```python
from build123d import *

# Parameters (mm, degrees)
CYLINDER1887_R     = 5
CYLINDER1887_DEPTH = 5
CYLINDER1886_R     = 2.5
CYLINDER1886_DEPTH = 40
CYLINDER1800_R     = 5
CYLINDER1800_DEPTH = 3
CYLINDER1801_R     = 2.5
CYLINDER1801_DEPTH = 20
CYLINDER1798_R     = 1.5
CYLINDER1798_DEPTH = 20
CYLINDER1796_R     = 1.5
CYLINDER1796_DEPTH = 20
CYLINDER1797_R     = 1.5
CYLINDER1797_DEPTH = 20
CYLINDER1799_R     = 1.5
CYLINDER1799_DEPTH = 20
BOX758_W           = 6
BOX758_H           = 6
BOX758_DEPTH       = 2
BOX760_W           = 6
BOX760_H           = 6
BOX760_DEPTH       = 2
BOX759_W           = 6
BOX759_H           = 6
BOX759_DEPTH       = 2
BOX756_W           = 6
BOX756_H           = 6
BOX756_DEPTH       = 2
BOX757_W           = 20
BOX757_H           = 80
BOX757_DEPTH       = 20
BOX761_W           = 38
BOX761_H           = 32
BOX761_DEPTH       = 26
CHAMFER064_SIZE    = 2


with BuildPart() as obj1:
    # Cylinder1887 → Cylinder1887 (new body)
    with BuildSketch(Plane(origin=(-86, 16, 68), x_dir=(0, 0, -1), z_dir=(1, 0, 0))):
        Circle(CYLINDER1887_R)
    extrude(amount=CYLINDER1887_DEPTH)


with BuildPart() as obj2:
    # Cylinder1886 → Cylinder1886 (new body)
    with BuildSketch(Plane(origin=(-90, 16, 68), x_dir=(0, 0, -1), z_dir=(1, 0, 0))):
        Circle(CYLINDER1886_R)
    extrude(amount=CYLINDER1886_DEPTH)


with BuildPart() as obj3:
    # Cylinder1800 → Cylinder1800 (new body)
    with BuildSketch(Plane(origin=(-112, 16, 66), x_dir=(0, 0, -1), z_dir=(1, 0, 0))):
        Circle(CYLINDER1800_R)
    extrude(amount=CYLINDER1800_DEPTH)


with BuildPart() as obj4:
    # Cylinder1801 → Cylinder1801 (new body)
    with BuildSketch(Plane(origin=(-117, 16, 66), x_dir=(0, 0, -1), z_dir=(1, 0, 0))):
        Circle(CYLINDER1801_R)
    extrude(amount=CYLINDER1801_DEPTH)


with BuildPart() as obj5:
    # Cylinder1798 → Cylinder1798 (new body)
    with BuildSketch(Plane(origin=(-83, 25, 54), x_dir=(1, 0, 0), z_dir=(0, 0, 1))):
        Circle(CYLINDER1798_R)
    extrude(amount=CYLINDER1798_DEPTH)


with BuildPart() as obj6:
    # Cylinder1796 → Cylinder1796 (new body)
    with BuildSketch(Plane(origin=(-109, 7, 54), x_dir=(1, 0, 0), z_dir=(0, 0, 1))):
        Circle(CYLINDER1796_R)
    extrude(amount=CYLINDER1796_DEPTH)


with BuildPart() as obj7:
    # Cylinder1797 → Cylinder1797 (new body)
    with BuildSketch(Plane(origin=(-109, 25, 54), x_dir=(1, 0, 0), z_dir=(0, 0, 1))):
        Circle(CYLINDER1797_R)
    extrude(amount=CYLINDER1797_DEPTH)


with BuildPart() as compound920:
    # Cylinder1799 → Cylinder1799 (new body)
    with BuildSketch(Plane(origin=(-83, 7, 54), x_dir=(1, 0, 0), z_dir=(0, 0, 1))):
        Circle(CYLINDER1799_R)
    extrude(amount=CYLINDER1799_DEPTH)

    # Compound920: union obj5, obj6, obj7
    add(obj5.part)
    add(obj6.part)
    add(obj7.part)


with BuildPart() as krychle758:
    # Box758 → Box758 (new body)
    with BuildSketch(Plane(origin=(-112, 22, 60), x_dir=(1, 0, 0), z_dir=(0, 0, 1))):
        with Locations((3, 3)):
            Rectangle(BOX758_W, BOX758_H)
    extrude(amount=BOX758_DEPTH)


with BuildPart() as krychle760:
    # Box760 → Box760 (new body)
    with BuildSketch(Plane(origin=(-86, 4, 60), x_dir=(1, 0, 0), z_dir=(0, 0, 1))):
        with Locations((3, 3)):
            Rectangle(BOX760_W, BOX760_H)
    extrude(amount=BOX760_DEPTH)


with BuildPart() as krychle759:
    # Box759 → Box759 (new body)
    with BuildSketch(Plane(origin=(-86, 22, 60), x_dir=(1, 0, 0), z_dir=(0, 0, 1))):
        with Locations((3, 3)):
            Rectangle(BOX759_W, BOX759_H)
    extrude(amount=BOX759_DEPTH)


with BuildPart() as compound918:
    # Box756 → Box756 (new body)
    with BuildSketch(Plane(origin=(-112, 4, 60), x_dir=(1, 0, 0), z_dir=(0, 0, 1))):
        with Locations((3, 3)):
            Rectangle(BOX756_W, BOX756_H)
    extrude(amount=BOX756_DEPTH)

    # Compound918: union Krychle758, Krychle760, Krychle759
    add(krychle758.part)
    add(krychle760.part)
    add(krychle759.part)


with BuildPart() as krychle757:
    # Box757 → Box757 (new body)
    with BuildSketch(Plane(origin=(-106, 4, 56), x_dir=(1, 0, 0), z_dir=(0, 0, 1))):
        with Locations((10, 40)):
            Rectangle(BOX757_W, BOX757_H)
    extrude(amount=BOX757_DEPTH)


with BuildPart() as cut620:
    # Box761 → Box761 (new body)
    with BuildSketch(Plane(origin=(-112, 0, 56), x_dir=(1, 0, 0), z_dir=(0, 0, 1))):
        with Locations((19, 16)):
            Rectangle(BOX761_W, BOX761_H)
    extrude(amount=BOX761_DEPTH)

    # Cut567: cut Krychle757
    add(krychle757.part, mode=Mode.SUBTRACT)

    # Cut569: cut Compound918
    add(compound918.part, mode=Mode.SUBTRACT)

    # Cut563: cut Compound920
    add(compound920.part, mode=Mode.SUBTRACT)

    # Cut564: cut obj4
    add(obj4.part, mode=Mode.SUBTRACT)

    # Cut560: cut obj3
    add(obj3.part, mode=Mode.SUBTRACT)

    # Chamfer064
    chamfer064_edges = [cut620.edges().sort_by_distance(p)[0] for p in [
        (-112, 32, 69),
    ]]
    chamfer(chamfer064_edges, length=CHAMFER064_SIZE)


with BuildPart() as cut620_1:
    # Chamfer064 placement: moved
    add(cut620.part.moved(Location((0, 0, 2))))

    # Cut619: cut obj2
    add(obj2.part, mode=Mode.SUBTRACT)

    # Cut620: cut obj1
    add(obj1.part, mode=Mode.SUBTRACT)


solid = cut620_1.part
```
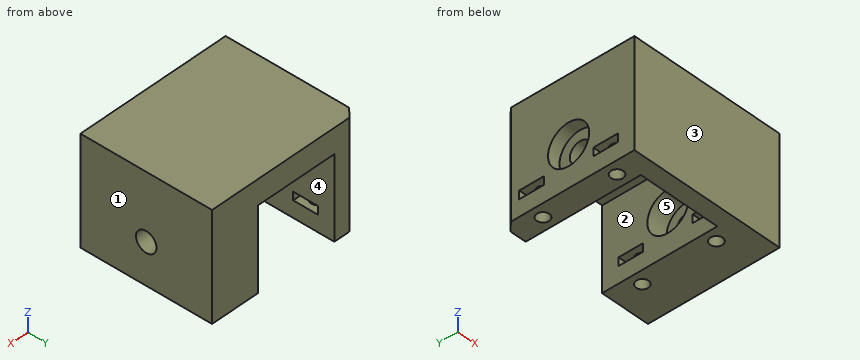
Can you work these out from the model? Positions are in its coordinate system, mm. Face numbers are marked on the shaded views. A direction names the side the tool comes from. Coordinates: 2 decimals unless noted, no trailing zeros. Write each loop counter-clockwise with the first axis right and the second up, starting at its lowest first coordinate (ties: lowest second). Pieces come first, ordered by that corner, then holes. Notation, with made-up numbers: M -11,-27.75 L 10,-27.75 A21 ccw 10,4.25 Z; hole C 72,-33 d1. An arc over 180 degrees is marked long. Write item = value, one per line. Start each with the question number.
Q1. If we section it at A-A, the plane y = 7: State how many separate pieces and enclosed holes the cut face has, then the cut area to 3 significant figures.
Q2. If I drill on L1, parallel to X at y = 25, z = 66.75; L2, parallel to Y at x = -83, z = 60.4; L3, parallel to Y at x = -83, z = 68.25, over which ranges is the centre line in solid material (lowest first)? Write a range as [from, to].
Q3. If we section it at C-C, the plane y = 16: Write out the boundary of the cut face in (x, z).
Q4. I'm going to push flat-ended pins straight in: pin 1 (10 mm diameter, centred on x = -95, z = 71.5, fed in from +Y); pin 2 (0.9 mm diameter, centred on x = -108.5, y = 25.5, fed in from -Z); pin 3 (1.5 mm diameter, centred on x = -88, y = 14.5, fed in from -Z). Where does each tip first touch, or does it pass through?
Q5. Thinking about a two-plate mould opening in Y: for the marked faces 3, 4 and 5, which applies, released by +Y, released by -Y, zero draft, split by the parting line, or undercut?
Q6. On a 3-axis mill with a long thin cutter (end or side, diameter ignored), from which of +Z, -Z, +X, -X, +Y, -Y can I reach the whole of each face in a straight line? I mean the marked faces 1 and 2. Say none if no direction works.
Check sheet entries:
q1.separate_pieces = 4
q1.enclosed_holes = 0
q1.area = 468 mm²
q2.L1 = [-112, -110.5], [-107.5, -106], [-86, -84.5], [-81.5, -74]
q2.L2 = [0, 5.5], [8.5, 23.5], [26.5, 32]
q2.L3 = [0, 5.5], [8.5, 11.01], [20.99, 23.5], [26.5, 32]
q3.outline = M -112,58 L -106,58 L -106,65.5 L -109,65.5 L -109,63 L -112,63 Z; M -112,73 L -109,73 L -109,70.5 L -106,70.5 L -106,78 L -86,78 L -86,73 L -81,73 L -81,70.5 L -74,70.5 L -74,84 L -112,84 Z; M -86,58 L -74,58 L -74,65.5 L -81,65.5 L -81,63 L -86,63 Z
q4.pin_1 = 4
q4.pin_2 = 76
q4.pin_3 = 78
q5.face_3 = released by -Y
q5.face_4 = zero draft
q5.face_5 = undercut
q6.face_1 = +Z, -Z, +X, +Y, -Y
q6.face_2 = -Z, +Y
